Geometry check sheet. Reference: the model listing, model coordinates, mm. A direction names the side the tool comes from. Coordinates: 2 decimals unless noted, no trailing zeros. Loops run counter-clockwise (first coordinate to the right, second up) from the corner with the lowest first, then second, coordinate; pieces in that order, holes last. Notation, with made-up numbers: (63, -9) - (71, -9) arc R8 ccw to (71, 6) - close; hole circle Ø4 at (7.25, 55). An arc over 180 degrees is marked (long way). Write each question's results on one line, items separated by ' | '. Start each with the question number.
(1) Access from +Z, -Z, +X, -X, +Y, -Y to the whole of each face (thin tool, end or side, straight path). Record for faces 1 (the face through (25, 31, 2)), 2 (the face through (41.93, 80.45, -0.03)), 3 (the face through (40.837, 63.913, 0.028)).
(2) Material ranges on probe 1 along X at (y, z) = (0, -0.7); probe 2 along Y at (x, z) = (24.5, 0.2); probe 3 along Y at (x, z) = (80, -0.8), recorded low to high.
(3) Go/stop test with a flat-tipped pin: pin 1 Ø1.5 at (y, z) = (103, 1.5) entering from +X. Record where the tip stops, or that it passes through.
(4) Sectioned sample at C-C (x = 45). Enter the section's corners in (y, z), plus the area to 3 significant figures.
(5) Sectioned sample at D-D (y = 97). Enter the section's corners in (x, z), plus the area to 3 significant figures.
(6) Sectioned sample at B-B (y = 0). Enter the section's corners in (x, z).
(7) Mould release check, pull along Y, two halves, no side actions. Record for faces 4 (the face through (-8.51, -5.25, 0.03)), 5 (the face through (39, -10, 0)), 6 (the face through (22.885, 14.746, 0.028)): pulls with the +Y half, pulls with the -Y half, needs draft (parallel to the pull), parting line crosses it, or undercut.
(8) Sectioned sample at A-A (z = -1.25). Enter the section's corners in (x, y).
from build123d import *

# Parameters (mm, degrees)
BOSS_EXTRUDE1_DEPTH     = 2
CUT_EXTRUDE1_DEPTH      = 150.177687816
CUT_EXTRUDE1_DEPTH_BACK = 150.177687816
CUT_EXTRUDE2_DEPTH      = 150.177687816
CUT_EXTRUDE2_DEPTH_BACK = 150.177687816
SKETCH4_R               = 4
FILLET2_R               = 10


with BuildPart() as part:
    # Sketch2 → Boss-Extrude1 (new, symmetric)
    with BuildSketch(Plane.XY):
        with BuildLine():
            ThreePointArc((0, 10), (-5.372996083, 8.433914458), (-9.06307787, 4.226182617))
            ThreePointArc((-9.06307787, 4.226182617), (-8.433914458, -5.372996083), (0, -10))
            ThreePointArc((0, -10), (5.372996083, -8.433914458), (9.06307787, -4.226182617))
            Line((9.06307787, -4.226182617), (15.696855771, 10))
            Line((15.696855771, 10), (0, 10))
        make_face()
        with BuildLine():
            Line((41.742866429, 113.179881771), (-9.06307787, 4.226182617))
            ThreePointArc((-9.06307787, 4.226182617), (-5.372996083, 8.433914458), (0, 10))
            Line((0, 10), (15.696855771, 10))
            Line((15.696855771, 10), (59.86902217, 104.727516536))
            ThreePointArc((59.86902217, 104.727516536), (55.032126917, 118.016777024), (41.742866429, 113.179881771))
        make_face()
        with BuildLine():
            ThreePointArc((9.06307787, -4.226182617), (5.372996083, -8.433914458), (0, -10))
            Line((0, -10), (80, -10))
            ThreePointArc((80, -10), (90, 0), (80, 10))
            Line((80, 10), (15.696855771, 10))
            Line((15.696855771, 10), (9.06307787, -4.226182617))
        make_face()
    extrude(amount=BOSS_EXTRUDE1_DEPTH, both=True)

    # Sketch3 → Cut-Extrude1 (cut, two sides: drawn at the far end of the back side and taken through both)
    with BuildSketch(Plane.XY.offset(-CUT_EXTRUDE1_DEPTH_BACK)):
        with BuildLine():
            Line((54.431175448, 107.263226106), (29.074079743, 52.884758884))
            ThreePointArc((29.074079743, 52.884758884), (23.758375548, 50.950000783), (21.823617447, 56.265704978))
            Line((21.823617447, 56.265704978), (47.180713151, 110.6441722))
            ThreePointArc((47.180713151, 110.6441722), (52.496417346, 112.578930301), (54.431175448, 107.263226106))
        make_face()
    extrude(amount=CUT_EXTRUDE1_DEPTH + CUT_EXTRUDE1_DEPTH_BACK, mode=Mode.SUBTRACT)

    # Sketch4 → Cut-Extrude2 (cut, two sides: drawn at the far end of the back side and taken through both)
    with BuildSketch(Plane.XY.offset(-CUT_EXTRUDE2_DEPTH_BACK)):
        with Locations((80, 0)):
            Circle(SKETCH4_R)
        Circle(SKETCH4_R)
    extrude(amount=CUT_EXTRUDE2_DEPTH + CUT_EXTRUDE2_DEPTH_BACK, mode=Mode.SUBTRACT)

    # Fillet2
    fillet2_edges = [part.edges().sort_by_distance(p)[0] for p in [
        (15.696855771, 10, 0),
    ]]
    fillet(fillet2_edges, radius=FILLET2_R)


solid = part.part
Outcome:
1) face 1: +Z, +X, -X, +Y, -Y | face 2: +Z, -Z | face 3: +Z, -Z, +X
2) probe 1: x = -10 to -4, 4 to 76, 84 to 90 | probe 2: y = -10 to 12.76, 28.88 to 50.69, 62.01 to 76.2 | probe 3: y = -10 to -4, 4 to 10
3) pin 1: stops at x = 59.41
4) outline: (-10, -2) - (10, -2) - (10, 2) - (-10, 2) - close; (72.84, -2) - (87.04, -2) - (87.04, 2) - (72.84, 2) - close; (105.97, -2) - (117.1, -2) - (117.1, 2) - (105.97, 2) - close | area: 181 mm2
5) outline: (34.2, -2) - (40.82, -2) - (40.82, 2) - (34.2, 2) - close; (49.65, -2) - (56.27, -2) - (56.27, 2) - (49.65, 2) - close | area: 53.0 mm2
6) outline: (-10, -2) - (-4, -2) - (-4, 2) - (-10, 2) - close; (4, -2) - (76, -2) - (76, 2) - (4, 2) - close; (84, -2) - (90, -2) - (90, 2) - (84, 2) - close
7) face 4: parting line crosses it | face 5: pulls with the -Y half | face 6: undercut
8) outline: (-9.06, 4.23) arc R10 ccw to (0, -10) - (80, -10) arc R10 ccw to (80, 10) - (31.39, 10) arc R10 cw to (22.33, 24.23) - (59.87, 104.73) arc R10 ccw to (41.74, 113.18) - close; hole circle Ø8 at (0, 0); hole (21.82, 56.27) arc R4 ccw to (29.07, 52.88) - (54.43, 107.26) arc R4 ccw to (47.18, 110.64) - close; hole circle Ø8 at (80, 0)
